Check sheet for the modelled part. Datum: model origin and axes. Units: mm. A direction names the side the tool comes from. Round coordinates to 2 decimals unless told otherwise and drop trailing zeros. Loops run counter-clockwise (first coordinate to the right, second up) from the corner with the lowest first, then second, coordinate; pieces in that order, holes last. Notation, with made-up numbers: (-19, 66) - (16, 66) arc R9 cw to (16, 81) - close; hole circle Ø9 at (33.5, 78.25). An arc over 180 degrees is marked (long way). Put each result on its own line as item: value.
```python
from build123d import *

# Parameters (mm, degrees)
SKETCH1_W           = 146.05
SKETCH1_H           = 101.6
BOSS_EXTRUDE1_DEPTH = 11.1125
BOSS_EXTRUDE2_START = -36.5125
SKETCH2_W           = 25.4
SKETCH2_H           = 101.6
BOSS_EXTRUDE2_DEPTH = 25.4
FILLET1_R           = 1.524
CUT_EXTRUDE2_START  = 11.1125
SKETCH3_R           = 19.4437
CUT_EXTRUDE2_DEPTH  = 36.5125
CUT_EXTRUDE4_START  = 11.1125
SKETCH4_R           = 6.7437
CUT_EXTRUDE4_DEPTH  = 108.270980028
CUT_EXTRUDE6_START  = 11.1125
SKETCH5_R           = 12.7
CUT_EXTRUDE6_DEPTH  = 14.2875
CUT_EXTRUDE8_START  = 11.1125
SKETCH6_R           = 5.1562
CUT_EXTRUDE8_DEPTH  = 108.270980028
CUT_EXTRUDE10_START = 11.1125
SKETCH7_R           = 7.9375
CUT_EXTRUDE10_DEPTH = 9.525
CUT_EXTRUDE12_START = 11.1125
SKETCH8_R           = 5.1562
CUT_EXTRUDE12_DEPTH = 108.270980028
CUT_EXTRUDE14_START = 11.1125
SKETCH9_R           = 7.9375
CUT_EXTRUDE14_DEPTH = 9.525
CUT_EXTRUDE16_START = 73.025
SKETCH10_R          = 5.1562
CUT_EXTRUDE16_DEPTH = 170.183480028
CUT_EXTRUDE18_START = 73.025
SKETCH11_R          = 7.9375
CUT_EXTRUDE18_DEPTH = 9.525


with BuildPart() as part:
    # Sketch1 → Boss-Extrude1 (new, symmetric)
    with BuildSketch(Plane(origin=(0, 0, 0), x_dir=(1, 0, 0), z_dir=(0, 1, 0))):
        Rectangle(SKETCH1_W, SKETCH1_H)
    extrude(amount=BOSS_EXTRUDE1_DEPTH, both=True)

    # Sketch2 → Boss-Extrude2 (add)
    with BuildSketch(Plane(origin=(0, 0, 0), x_dir=(1, 0, 0), z_dir=(0, 1, 0)).offset(BOSS_EXTRUDE2_START)):
        with Locations((60.325, 0)):
            Rectangle(SKETCH2_W, SKETCH2_H)
    extrude(amount=BOSS_EXTRUDE2_DEPTH)

    # Fillet1
    fillet1_edges = [part.edges().sort_by_distance(p)[0] for p in [
        (47.625, -11.1125, 0),
    ]]
    fillet(fillet1_edges, radius=FILLET1_R)

    # Sketch3 → Cut-Extrude2 (cut)
    with BuildSketch(Plane(origin=(0, 0, 0), x_dir=(1, 0, 0), z_dir=(0, 1, 0)).offset(CUT_EXTRUDE2_START)):
        with Locations(Location((-31.75, 0, 0), (0, 0, 270))):
            Circle(SKETCH3_R)
    extrude(amount=-CUT_EXTRUDE2_DEPTH, mode=Mode.SUBTRACT)

    # Sketch4 → Cut-Extrude4 (cut, through all)
    with BuildSketch(Plane(origin=(0, 0, 0), x_dir=(1, 0, 0), z_dir=(0, 1, 0)).offset(CUT_EXTRUDE4_START)):
        with Locations(Location((-57.785, -26.035, 0), (0, 0, 270))):
            Circle(SKETCH4_R)
        with Locations(Location((-5.715, -26.035, 0), (0, 0, 270))):
            Circle(SKETCH4_R)
        with Locations(Location((-57.785, 26.035, 0), (0, 0, 270))):
            Circle(SKETCH4_R)
        with Locations(Location((-5.715, 26.035, 0), (0, 0, 270))):
            Circle(SKETCH4_R)
    extrude(amount=-CUT_EXTRUDE4_DEPTH, mode=Mode.SUBTRACT)

    # Sketch5 → Cut-Extrude6 (cut)
    with BuildSketch(Plane(origin=(0, 0, 0), x_dir=(1, 0, 0), z_dir=(0, 1, 0)).offset(CUT_EXTRUDE6_START)):
        with Locations(Location((-57.785, -26.035, 0), (0, 0, 270))):
            Circle(SKETCH5_R)
        with Locations(Location((-5.715, -26.035, 0), (0, 0, 270))):
            Circle(SKETCH5_R)
        with Locations(Location((-57.785, 26.035, 0), (0, 0, 270))):
            Circle(SKETCH5_R)
        with Locations(Location((-5.715, 26.035, 0), (0, 0, 270))):
            Circle(SKETCH5_R)
    extrude(amount=-CUT_EXTRUDE6_DEPTH, mode=Mode.SUBTRACT)

    # Sketch6 → Cut-Extrude8 (cut, through all)
    with BuildSketch(Plane(origin=(0, 0, 0), x_dir=(1, 0, 0), z_dir=(0, 1, 0)).offset(CUT_EXTRUDE8_START)):
        with Locations(Location((38.1, -38.1, 0), (0, 0, 270))):
            Circle(SKETCH6_R)
        with Locations(Location((38.1, 38.1, 0), (0, 0, 270))):
            Circle(SKETCH6_R)
    extrude(amount=-CUT_EXTRUDE8_DEPTH, mode=Mode.SUBTRACT)

    # Sketch7 → Cut-Extrude10 (cut)
    with BuildSketch(Plane(origin=(0, 0, 0), x_dir=(1, 0, 0), z_dir=(0, 1, 0)).offset(CUT_EXTRUDE10_START)):
        with Locations(Location((38.1, -38.1, 0), (0, 0, 270))):
            Circle(SKETCH7_R)
        with Locations(Location((38.1, 38.1, 0), (0, 0, 270))):
            Circle(SKETCH7_R)
    extrude(amount=-CUT_EXTRUDE10_DEPTH, mode=Mode.SUBTRACT)

    # Sketch8 → Cut-Extrude12 (cut, through all)
    with BuildSketch(Plane(origin=(0, 0, 0), x_dir=(1, 0, 0), z_dir=(0, 1, 0)).offset(CUT_EXTRUDE12_START)):
        with Locations(Location((22.225, 0, 0), (0, 0, 270))):
            Circle(SKETCH8_R)
    extrude(amount=-CUT_EXTRUDE12_DEPTH, mode=Mode.SUBTRACT)

    # Sketch9 → Cut-Extrude14 (cut)
    with BuildSketch(Plane(origin=(0, 0, 0), x_dir=(1, 0, 0), z_dir=(0, 1, 0)).offset(CUT_EXTRUDE14_START)):
        with Locations(Location((22.225, 0, 0), (0, 0, 270))):
            Circle(SKETCH9_R)
    extrude(amount=-CUT_EXTRUDE14_DEPTH, mode=Mode.SUBTRACT)

    # Sketch10 → Cut-Extrude16 (cut, through all)
    with BuildSketch(Plane(origin=(0, 0, 0), x_dir=(0, 0, -1), z_dir=(1, 0, 0)).offset(CUT_EXTRUDE16_START)):
        with Locations((-22.225, -23.8125)):
            Circle(SKETCH10_R)
        with Locations((22.225, -23.8125)):
            Circle(SKETCH10_R)
    extrude(amount=-CUT_EXTRUDE16_DEPTH, mode=Mode.SUBTRACT)

    # Sketch11 → Cut-Extrude18 (cut)
    with BuildSketch(Plane(origin=(0, 0, 0), x_dir=(0, 0, -1), z_dir=(1, 0, 0)).offset(CUT_EXTRUDE18_START)):
        with Locations((-22.225, -23.8125)):
            Circle(SKETCH11_R)
        with Locations((22.225, -23.8125)):
            Circle(SKETCH11_R)
    extrude(amount=-CUT_EXTRUDE18_DEPTH, mode=Mode.SUBTRACT)


solid = part.part
```
Item 1: Section check D-D on x = -24. Enter the section's corners in (y, z).
Filled sheet:
outline: (-11.11, -50.8) - (11.11, -50.8) - (11.11, -17.83) - (-11.11, -17.83) - close; (-11.11, 17.83) - (11.11, 17.83) - (11.11, 50.8) - (-11.11, 50.8) - close
Item 2: Release check for a two-part mould opening along Z. For faces 1 (the cylindrical face through (55.67, -28.39, 19.85)), 2 (the flat face through (36, 1.588, -33)), 3 (the flat face through (60, -36.512, -1)), 4 (the flat face through (15, -2, -50.8)) record: +Z half, -Z half, draft (parallel to the pull), parting line (faces both ways), or undercut.
Filled sheet:
face 1: undercut
face 2: undercut
face 3: draft
face 4: -Z half
Item 3: Thickness scan on line 1 (Z direction, x = -58.5, y = -3); line 2 (Z direction, x = 38, y = 5); line 3 (X direction, y = -4.5, z = -30.5) (3 decimals). Record the ranges inside material, lowest first. Write a range as from..to.
Filled sheet:
line 1: -50.8..-38.71, -13.36..13.36, 38.71..50.8
line 2: -50.8..-46.04, -30.16..30.16, 46.04..50.8
line 3: -73.025..-62.839, -52.731..-10.769, -0.661..73.025
Item 4: Section check B-B on z = 0. Enter the section's corners in (x, y) (1 decimal), then the cut area to 3 significant figures.
Filled sheet:
outline: (-73, -11.1) - (-51.2, -11.1) - (-51.2, 11.1) - (-73, 11.1) - close; (-12.3, -11.1) - (17.1, -11.1) - (17.1, 1.6) - (14.3, 1.6) - (14.3, 11.1) - (-12.3, 11.1) - close; (27.4, -11.1) - (46.1, -11.1) arc R1.5 cw to (47.6, -12.6) - (47.6, -36.5) - (73, -36.5) - (73, 11.1) - (30.2, 11.1) - (30.2, 1.6) - (27.4, 1.6) - close
area: 2,750 mm²
Item 5: Section check C-C on y = -1.5. Count the separate pieces of the cut face and the enclosed holes in it, then the cut area to 3 significant figures.
Filled sheet:
separate pieces: 1
enclosed holes: 8
area: 11,400 mm²
Item 6: Go/stop test with flat-tipped pins: pin 1 (7.5 mm diameter, centred on x = -8.5, z = 29.5, fed in from +Y) (3 decimals); pin 2 (12 mm diameter, centred on y = -27.5, z = 13.5, fed in from -X) (3 decimals); pin 3 (8 mm diameter, centred on x = 40, z = -41.5, fed in from +Y). Record where each tip stops, or that it passes through.
Filled sheet:
pin 1: y = -3.175
pin 2: x = 47.625
pin 3: y = 1.59
Item 7: Section check A-A on x = 38.1. Enter the section's corners in (y, z).
Filled sheet:
outline: (-11.11, -50.8) - (11.11, -50.8) - (11.11, -46.04) - (1.59, -46.04) - (1.59, -43.26) - (-11.11, -43.26) - close; (-11.11, -32.94) - (1.59, -32.94) - (1.59, -30.16) - (11.11, -30.16) - (11.11, 30.16) - (1.59, 30.16) - (1.59, 32.94) - (-11.11, 32.94) - close; (-11.11, 43.26) - (1.59, 43.26) - (1.59, 46.04) - (11.11, 46.04) - (11.11, 50.8) - (-11.11, 50.8) - close
Item 8: Tool access check on faces 5 (the flat face through (-63, -3.175, -21)), 6 (the cylindrical face through (68.329, -23.464, 30.155)), 7 (the cylindrical face through (34.96, -4.67, 34.01)). Record the directions out of +Z, -Z, +X, -X, +Y, -Y that give a thin tool (end or side, any length) a straight path to the whole face; none if there is none.
Filled sheet:
face 5: +Y
face 6: +X
face 7: +Y, -Y
